```python
from build123d import *

# Parameters (mm, degrees)
F0_R      = 5
F1_DEPTH  = 6
F2_DEPTH  = 5
F3_DEPTH  = 3.1
F6_R      = 10
F6_R_2    = 3.5
F7_DEPTH  = 2
F8_R      = 10
F8_R_2    = 5.25
F9_DEPTH  = 1.125
F11_DEPTH = 2.125


with BuildPart() as f1:
    # F0 (on Top) → F1 (new body)
    with BuildSketch(Plane.XY):
        Circle(F0_R)
        with BuildLine():
            ThreePointArc((0.75, 2.4372115214), (2.0512191497, 1.5149257408), (2.55, 0))
            ThreePointArc((2.55, 0), (2.0512191497, -1.5149257408), (0.75, -2.4372115214))
            ThreePointArc((0.75, -2.4372115214), (0, -2.55), (-0.75, -2.4372115214))
            ThreePointArc((-0.75, -2.4372115214), (-2.55, 0), (-0.75, 2.4372115214))
            ThreePointArc((-0.75, 2.4372115214), (0, 2.55), (0.75, 2.4372115214))
        make_face(mode=Mode.SUBTRACT)
    extrude(amount=F1_DEPTH)

    # F0 (on Top) → F2 (join)
    with BuildSketch(Plane.XY):
        with BuildLine():
            Line((0.75, 1.2990381057), (0.75, 2.4372115214))
            ThreePointArc((0.75, 2.4372115214), (0, 2.55), (-0.75, 2.4372115214))
            Line((-0.75, 2.4372115214), (-0.75, 1.2990381057))
            ThreePointArc((-0.75, 1.2990381057), (0, 1.5), (0.75, 1.2990381057))
        make_face()
        with BuildLine():
            ThreePointArc((-0.75, -2.4372115214), (0, -2.55), (0.75, -2.4372115214))
            Line((0.75, -2.4372115214), (0.75, -1.2990381057))
            ThreePointArc((0.75, -1.2990381057), (0, -1.5), (-0.75, -1.2990381057))
            Line((-0.75, -1.2990381057), (-0.75, -2.4372115214))
        make_face()
    extrude(amount=F2_DEPTH)

    # F0 (on Top) → F3 (join)
    with BuildSketch(Plane.XY):
        with BuildLine():
            Line((-0.75, 1.2990381057), (-0.75, 2.4372115214))
            ThreePointArc((-0.75, 2.4372115214), (-2.55, 0), (-0.75, -2.4372115214))
            Line((-0.75, -2.4372115214), (-0.75, -1.2990381057))
            ThreePointArc((-0.75, -1.2990381057), (-1.5, 0), (-0.75, 1.2990381057))
        make_face()
        with BuildLine():
            ThreePointArc((0.75, -2.4372115214), (2.0512191497, -1.5149257408), (2.55, 0))
            ThreePointArc((2.55, 0), (2.0512191497, 1.5149257408), (0.75, 2.4372115214))
            Line((0.75, 2.4372115214), (0.75, 1.2990381057))
            ThreePointArc((0.75, 1.2990381057), (1.2990381057, 0.75), (1.5, 0))
            ThreePointArc((1.5, 0), (1.2990381057, -0.75), (0.75, -1.2990381057))
            Line((0.75, -1.2990381057), (0.75, -2.4372115214))
        make_face()
    extrude(amount=F3_DEPTH)

    # F4 (on Front) → F5 (revolve)
    with BuildSketch(Plane.XZ):
        Polygon((-10, 0), (-4, 0), (-4, 5), (-4.5, 5), (-10, 3), align=None)
    revolve(axis=Axis((0, 0, 1.2425027974), (0, 0, 1)))

    # F6 (on face) → F7 (join)
    with BuildSketch(Plane(origin=(0, 0, 0), x_dir=(1, 0, 0), z_dir=(0, 0, -1))):
        Circle(F6_R)
        Circle(F6_R_2, mode=Mode.SUBTRACT)
    extrude(amount=F7_DEPTH)

    # F8 (on face) → F9 (join)
    with BuildSketch(Plane(origin=(0, 0, -2), x_dir=(1, 0, 0), z_dir=(0, 0, -1))):
        Circle(F8_R)
        Circle(F8_R_2, mode=Mode.SUBTRACT)
    extrude(amount=F9_DEPTH)

    # F10 (on face) → F11 (cut)
    with BuildSketch(Plane(origin=(0, 0, -3.125), x_dir=(1, 0, 0), z_dir=(0, 0, -1))):
        with BuildLine():
            ThreePointArc((-7, -2), (-5.5857864376, -1.4142135624), (-5, 0))
            ThreePointArc((-5, 0), (-5.5857864376, 1.4142135624), (-7, 2))
            ThreePointArc((-7, 2), (-9, 0), (-7, -2))
        make_face()
        with BuildLine():
            ThreePointArc((7, -2), (8.4142135624, -1.4142135624), (9, 0))
            ThreePointArc((9, 0), (8.4142135624, 1.4142135624), (7, 2))
            ThreePointArc((7, 2), (5, 0), (7, -2))
        make_face()
    extrude(amount=-F11_DEPTH, mode=Mode.SUBTRACT)


solid = f1.part
```
Model file for the job. Use its own axes, mm. A direction names the side the tool comes from. Give positions to 0.01 mm unless a question says otherwise; leave off trailing zeros. Write each loop counter-clockwise with the first axis right and the second up, starting at its lowest first coordinate (ties: lowest second). Pieces come first, ordered by that corner, then holes. Notation, with made-up numbers: (83, 50.5) -> (122, 50.5) arc R14 cw to (122, 58.5) -> close; hole circle Ø7 at (10, -13). An arc over 180 degrees is marked (long way). Use CSV: the item, a comma, the result in double quotes. Start each with the question number.
1) Pin check, flat tips, straight feed: P1, Ø5.5, axis at x = 0, y = 0, coming from the -Z side; P2, Ø1, axis at y = 4.5, z = 1.5, coming from the +X side; P3, Ø0.6, axis at x = 0, y = 2, coming from the +Z side. Stop position of each tip, or through.
2) Cut at A-A on x = 0. List the corners of the cut face in (y, z) (3 decimals), plus the area to 3 significant figures.
3) Drill centre lines: L1, parallel to Y at x = 0, z = -1.4; L2, parallel to Y at x = 2.5, z = -0.75. Where is each one in solid material? Low to high.
4) Tool access for faces 1 (the flat face through (4, 4, -3.125)), 2 (the cylindrical face through (-0.1, 5.25, -2.55)), 3 (the flat face through (0, -2, 5)): list every direction of +Z, -Z, +X, -X, +Y, -Y with a clear straight run to the whole face (end or side of a thin tool).
5) Cut at B-B on z = -0.25. List the corners of the cut face in (x, y).
6) Two-plate mould, pull along X, no slides. Class faces 4 (the flat face through (-0.75, 2, 4)), 5 (the cylindrical face through (-1.08, -4.88, 5.4)), 6 (the flat face through (2, -2, 6)): released by +X, released by -X, zero draft, split by the parting line, or undercut.
Final values:
1,P1,"stops at z = 0"
1,P2,"stops at x = 9.17"
1,P3,"stops at z = 5"
2,outline,"(-10, -3.125) -> (-5.25, -3.125) -> (-5.25, -2) -> (-3.5, -2) -> (-3.5, 0) -> (-1.5, 0) -> (-1.5, 5) -> (-2.55, 5) -> (-2.55, 6) -> (-5, 6) -> (-5, 4.818) -> (-10, 3) -> close; (1.5, 0) -> (3.5, 0) -> (3.5, -2) -> (5.25, -2) -> (5.25, -3.125) -> (10, -3.125) -> (10, 3) -> (5, 4.818) -> (5, 6) -> (2.55, 6) -> (2.55, 5) -> (1.5, 5) -> close"
2,area,"116 mm2"
3,L1,"y = -10 to -3.5, 3.5 to 10"
3,L2,"y = -9.68 to -2.45, 2.45 to 9.68"
4,face 1,"-Z, +X, -X, +Y, -Y"
4,face 2,"-Z"
4,face 3,"+Z"
5,outline,"circle Ø20 at (0, 0); hole circle Ø7 at (0, 0)"
6,face 4,"undercut"
6,face 5,"split by the parting line"
6,face 6,"zero draft"
